from build123d import *

# Parameters (mm, degrees)
SKETCH2_W                 = 230
SKETCH2_H                 = 40
BOSS_EXTRUDE1_DEPTH       = 80
SKETCH6_R                 = 25
BOSS_EXTRUDE3_DEPTH       = 50
SKETCH7_R                 = 12.5
CUT_EXTRUDE2_DEPTH        = 50
SKETCH8_R                 = 26.5
CUT_EXTRUDE3_DEPTH        = 25
CUT_EXTRUDE4_START        = 40
SKETCH11_R                = 26.5
CUT_EXTRUDE4_DEPTH        = 40
SKETCH14_W                = 12.614661349
SKETCH14_H                = 40
CUT_EXTRUDE6_DEPTH        = 50
FILLET3_R                 = 20
FILLET3_OF_MIRROR5_R      = 20
FILLET3_OF_MIRROR8_R      = 20
SKETCH15_W                = 230
SKETCH15_H                = 40
BOSS_EXTRUDE4_DEPTH       = 50
SKETCH18_W                = 206
SKETCH18_H                = 16
CUT_EXTRUDE7_DEPTH        = 80
SKETCH21_R                = 7.5
CUT_EXTRUDE8_DEPTH        = 5
SKETCH22_R                = 5
CUT_EXTRUDE9_DEPTH        = 35
LPATTERN1_COUNT           = 4
LPATTERN1_PITCH           = 17
MIRROR9_COPY_1_SKETCH_R   = 7.5
MIRROR9_COPY_1_DEPTH      = 5
MIRROR9_COPY_2_SKETCH_R   = 7.5
MIRROR9_COPY_2_DEPTH      = 5
MIRROR9_COPY_3_SKETCH_R   = 7.5
MIRROR9_COPY_3_DEPTH      = 5
MIRROR9_COPY_4_SKETCH_R   = 5
MIRROR9_COPY_4_DEPTH      = 35
MIRROR9_COPY_5_SKETCH_R   = 5
MIRROR9_COPY_5_DEPTH      = 35
MIRROR9_COPY_6_SKETCH_R   = 5
MIRROR9_COPY_6_DEPTH      = 35
MIRROR10_COPY_1_SKETCH_R  = 7.5
MIRROR10_COPY_1_DEPTH     = 5
MIRROR10_COPY_2_SKETCH_R  = 7.5
MIRROR10_COPY_2_DEPTH     = 5
MIRROR10_COPY_3_SKETCH_R  = 7.5
MIRROR10_COPY_3_DEPTH     = 5
MIRROR10_COPY_4_SKETCH_R  = 5
MIRROR10_COPY_4_DEPTH     = 35
MIRROR10_COPY_5_SKETCH_R  = 5
MIRROR10_COPY_5_DEPTH     = 35
MIRROR10_COPY_6_SKETCH_R  = 5
MIRROR10_COPY_6_DEPTH     = 35
MIRROR10_COPY_7_SKETCH_R  = 7.5
MIRROR10_COPY_7_DEPTH     = 5
MIRROR10_COPY_8_SKETCH_R  = 5
MIRROR10_COPY_8_DEPTH     = 35
MIRROR10_COPY_9_SKETCH_R  = 7.5
MIRROR10_COPY_9_DEPTH     = 5
MIRROR10_COPY_10_SKETCH_R = 7.5
MIRROR10_COPY_10_DEPTH    = 5
MIRROR10_COPY_11_SKETCH_R = 7.5
MIRROR10_COPY_11_DEPTH    = 5
MIRROR10_COPY_12_SKETCH_R = 5
MIRROR10_COPY_12_DEPTH    = 35
MIRROR10_COPY_13_SKETCH_R = 5
MIRROR10_COPY_13_DEPTH    = 35
MIRROR10_COPY_14_SKETCH_R = 5
MIRROR10_COPY_14_DEPTH    = 35


with BuildPart() as part:
    # Sketch2 → Boss-Extrude1 (new body)
    with BuildSketch(Plane.XY):
        with Locations((115, 20)):
            Rectangle(SKETCH2_W, SKETCH2_H)
    extrude(amount=BOSS_EXTRUDE1_DEPTH)

    # Sketch6 → Boss-Extrude3 (add)
    with BuildSketch(Plane(origin=(140, 0, 0), x_dir=(0, 0, -1), z_dir=(1, 0, 0))):
        with Locations((10, 20)):
            Circle(SKETCH6_R)
    boss_extrude3 = extrude(amount=BOSS_EXTRUDE3_DEPTH)

    # Sketch7 → Cut-Extrude2 (cut)
    with BuildSketch(Plane.ZY.offset(-140)):
        with Locations(Location((-10, 20, 0), (0, 0, 36.869897646))):
            Circle(SKETCH7_R)
    cut_extrude2 = extrude(amount=-CUT_EXTRUDE2_DEPTH, mode=Mode.SUBTRACT)

    # Sketch8 → Cut-Extrude3 (cut)
    with BuildSketch(Plane.ZY.offset(-140)):
        with Locations((-10, 20)):
            Circle(SKETCH8_R)
    cut_extrude3 = extrude(amount=CUT_EXTRUDE3_DEPTH, mode=Mode.SUBTRACT)

    # Sketch11 → Cut-Extrude4 (cut)
    with BuildSketch(Plane(origin=(190, 0, 0), x_dir=(0, 0, -1), z_dir=(1, 0, 0)).offset(CUT_EXTRUDE4_START)):
        with Locations((10, 20)):
            Circle(SKETCH11_R)
    cut_extrude4 = extrude(amount=-CUT_EXTRUDE4_DEPTH, mode=Mode.SUBTRACT)

    # Mirror1: Boss-Extrude3, Cut-Extrude2, Cut-Extrude3, Cut-Extrude4 across plane
    add(boss_extrude3.mirror(Plane(origin=(115, 0, 0), x_dir=(0, 0, 1), z_dir=(1, 0, 0))))
    add(cut_extrude2.mirror(Plane(origin=(115, 0, 0), x_dir=(0, 0, 1), z_dir=(1, 0, 0))), mode=Mode.SUBTRACT)
    add(cut_extrude3.mirror(Plane(origin=(115, 0, 0), x_dir=(0, 0, 1), z_dir=(1, 0, 0))), mode=Mode.SUBTRACT)
    add(cut_extrude4.mirror(Plane(origin=(115, 0, 0), x_dir=(0, 0, 1), z_dir=(1, 0, 0))), mode=Mode.SUBTRACT)

    # Sketch14 → Cut-Extrude6 (cut)
    with BuildSketch(Plane(origin=(90, 0, 0), x_dir=(0, 0, -1), z_dir=(1, 0, 0))):
        with Locations((-13.692669326, 20)):
            Rectangle(SKETCH14_W, SKETCH14_H)
    cut_extrude6 = extrude(amount=CUT_EXTRUDE6_DEPTH, mode=Mode.SUBTRACT)

    # Fillet3
    fillet3_edges = [part.edges().sort_by_distance(p)[0] for p in [
        (115, 40, 20),
        (115, 0, 20),
    ]]
    fillet(fillet3_edges, radius=FILLET3_R - 0.0001)  # a hair under: the kernel refuses the full size

    # Mirror5: Cut-Extrude6 across plane
    add(cut_extrude6.mirror(Plane.ZY.offset(-165)), mode=Mode.SUBTRACT)

    # Fillet3 of Mirror5
    fillet3_of_mirror5_edges = [part.edges().sort_by_distance(p)[0] for p in [
        (210, 40, 20),
        (210, 0, 20),
    ]]
    fillet(fillet3_of_mirror5_edges, radius=FILLET3_OF_MIRROR5_R - 0.0001)  # a hair under: the kernel refuses the full size

    # Mirror8: Cut-Extrude6 across plane
    add(cut_extrude6.mirror(Plane(origin=(65, 0, 0), x_dir=(0, 0, 1), z_dir=(1, 0, 0))), mode=Mode.SUBTRACT)

    # Fillet3 of Mirror8
    fillet3_of_mirror8_edges = [part.edges().sort_by_distance(p)[0] for p in [
        (20, 40, 20),
        (20, 0, 20),
    ]]
    fillet(fillet3_of_mirror8_edges, radius=FILLET3_OF_MIRROR8_R - 0.0001)  # a hair under: the kernel refuses the full size

    # Sketch15 → Boss-Extrude4 (add)
    with BuildSketch(Plane.XY.offset(80)):
        with Locations((115, 20)):
            Rectangle(SKETCH15_W, SKETCH15_H)
    extrude(amount=BOSS_EXTRUDE4_DEPTH)

    # Sketch18 → Cut-Extrude7 (cut)
    with BuildSketch(Plane.XY.offset(130)):
        with Locations((115, 20)):
            Rectangle(SKETCH18_W, SKETCH18_H)
    extrude(amount=-CUT_EXTRUDE7_DEPTH, mode=Mode.SUBTRACT)

    # Sketch21 → Cut-Extrude8 (cut)
    with BuildSketch(Plane(origin=(0, 40, 0), x_dir=(1, 0, 0), z_dir=(0, 1, 0))):
        with Locations(Location((37, -66, 0), (0, 0, 270))):
            Circle(SKETCH21_R)
    cut_extrude8 = extrude(amount=-CUT_EXTRUDE8_DEPTH, mode=Mode.SUBTRACT)

    # Sketch22 → Cut-Extrude9 (cut)
    with BuildSketch(Plane(origin=(0, 35, 0), x_dir=(1, 0, 0), z_dir=(0, 1, 0))):
        with Locations(Location((37, -66, 0), (0, 0, 270))):
            Circle(SKETCH22_R)
    cut_extrude9 = extrude(amount=-CUT_EXTRUDE9_DEPTH, mode=Mode.SUBTRACT)

    # LPattern1: Cut-Extrude8, Cut-Extrude9 ×4
    with Locations(*[(0, 0, i * LPATTERN1_PITCH) for i in range(1, LPATTERN1_COUNT)]):
        add(cut_extrude8, mode=Mode.SUBTRACT)
        add(cut_extrude9, mode=Mode.SUBTRACT)

    # Mirror9: Cut-Extrude8, Cut-Extrude9 across plane
    add(cut_extrude8.mirror(Plane(origin=(63.5, 0, 0), x_dir=(0, 0, 1), z_dir=(1, 0, 0))), mode=Mode.SUBTRACT)
    add(cut_extrude9.mirror(Plane(origin=(63.5, 0, 0), x_dir=(0, 0, 1), z_dir=(1, 0, 0))), mode=Mode.SUBTRACT)

    # Mirror9 copy 1 sketch → Mirror9 copy 1 (cut)
    with BuildSketch(Plane(origin=(127, 40, 17), x_dir=(-1, 0, 0), z_dir=(0, 1, 0))):
        with Locations((37, 66)):
            Circle(MIRROR9_COPY_1_SKETCH_R)
    extrude(amount=-MIRROR9_COPY_1_DEPTH, mode=Mode.SUBTRACT)

    # Mirror9 copy 2 sketch → Mirror9 copy 2 (cut)
    with BuildSketch(Plane(origin=(127, 40, 34), x_dir=(-1, 0, 0), z_dir=(0, 1, 0))):
        with Locations((37, 66)):
            Circle(MIRROR9_COPY_2_SKETCH_R)
    extrude(amount=-MIRROR9_COPY_2_DEPTH, mode=Mode.SUBTRACT)

    # Mirror9 copy 3 sketch → Mirror9 copy 3 (cut)
    with BuildSketch(Plane(origin=(127, 40, 51), x_dir=(-1, 0, 0), z_dir=(0, 1, 0))):
        with Locations((37, 66)):
            Circle(MIRROR9_COPY_3_SKETCH_R)
    extrude(amount=-MIRROR9_COPY_3_DEPTH, mode=Mode.SUBTRACT)

    # Mirror9 copy 4 sketch → Mirror9 copy 4 (cut)
    with BuildSketch(Plane(origin=(127, 35, 17), x_dir=(-1, 0, 0), z_dir=(0, 1, 0))):
        with Locations((37, 66)):
            Circle(MIRROR9_COPY_4_SKETCH_R)
    extrude(amount=-MIRROR9_COPY_4_DEPTH, mode=Mode.SUBTRACT)

    # Mirror9 copy 5 sketch → Mirror9 copy 5 (cut)
    with BuildSketch(Plane(origin=(127, 35, 34), x_dir=(-1, 0, 0), z_dir=(0, 1, 0))):
        with Locations((37, 66)):
            Circle(MIRROR9_COPY_5_SKETCH_R)
    extrude(amount=-MIRROR9_COPY_5_DEPTH, mode=Mode.SUBTRACT)

    # Mirror9 copy 6 sketch → Mirror9 copy 6 (cut)
    with BuildSketch(Plane(origin=(127, 35, 51), x_dir=(-1, 0, 0), z_dir=(0, 1, 0))):
        with Locations((37, 66)):
            Circle(MIRROR9_COPY_6_SKETCH_R)
    extrude(amount=-MIRROR9_COPY_6_DEPTH, mode=Mode.SUBTRACT)

    # Mirror10: Cut-Extrude8, Cut-Extrude9 across plane
    add(cut_extrude8.mirror(Plane(origin=(115, 0, 0), x_dir=(0, 0, 1), z_dir=(1, 0, 0))), mode=Mode.SUBTRACT)
    add(cut_extrude9.mirror(Plane(origin=(115, 0, 0), x_dir=(0, 0, 1), z_dir=(1, 0, 0))), mode=Mode.SUBTRACT)

    # Mirror10 copy 1 sketch → Mirror10 copy 1 (cut)
    with BuildSketch(Plane(origin=(230, 40, 17), x_dir=(-1, 0, 0), z_dir=(0, 1, 0))):
        with Locations((37, 66)):
            Circle(MIRROR10_COPY_1_SKETCH_R)
    extrude(amount=-MIRROR10_COPY_1_DEPTH, mode=Mode.SUBTRACT)

    # Mirror10 copy 2 sketch → Mirror10 copy 2 (cut)
    with BuildSketch(Plane(origin=(230, 40, 34), x_dir=(-1, 0, 0), z_dir=(0, 1, 0))):
        with Locations((37, 66)):
            Circle(MIRROR10_COPY_2_SKETCH_R)
    extrude(amount=-MIRROR10_COPY_2_DEPTH, mode=Mode.SUBTRACT)

    # Mirror10 copy 3 sketch → Mirror10 copy 3 (cut)
    with BuildSketch(Plane(origin=(230, 40, 51), x_dir=(-1, 0, 0), z_dir=(0, 1, 0))):
        with Locations((37, 66)):
            Circle(MIRROR10_COPY_3_SKETCH_R)
    extrude(amount=-MIRROR10_COPY_3_DEPTH, mode=Mode.SUBTRACT)

    # Mirror10 copy 4 sketch → Mirror10 copy 4 (cut)
    with BuildSketch(Plane(origin=(230, 35, 17), x_dir=(-1, 0, 0), z_dir=(0, 1, 0))):
        with Locations((37, 66)):
            Circle(MIRROR10_COPY_4_SKETCH_R)
    extrude(amount=-MIRROR10_COPY_4_DEPTH, mode=Mode.SUBTRACT)

    # Mirror10 copy 5 sketch → Mirror10 copy 5 (cut)
    with BuildSketch(Plane(origin=(230, 35, 34), x_dir=(-1, 0, 0), z_dir=(0, 1, 0))):
        with Locations((37, 66)):
            Circle(MIRROR10_COPY_5_SKETCH_R)
    extrude(amount=-MIRROR10_COPY_5_DEPTH, mode=Mode.SUBTRACT)

    # Mirror10 copy 6 sketch → Mirror10 copy 6 (cut)
    with BuildSketch(Plane(origin=(230, 35, 51), x_dir=(-1, 0, 0), z_dir=(0, 1, 0))):
        with Locations((37, 66)):
            Circle(MIRROR10_COPY_6_SKETCH_R)
    extrude(amount=-MIRROR10_COPY_6_DEPTH, mode=Mode.SUBTRACT)

    # Mirror10 copy 7 sketch → Mirror10 copy 7 (cut)
    with BuildSketch(Plane(origin=(103, 40, 0), x_dir=(1, 0, 0), z_dir=(0, 1, 0))):
        with Locations(Location((37, -66, 0), (0, 0, 270))):
            Circle(MIRROR10_COPY_7_SKETCH_R)
    extrude(amount=-MIRROR10_COPY_7_DEPTH, mode=Mode.SUBTRACT)

    # Mirror10 copy 8 sketch → Mirror10 copy 8 (cut)
    with BuildSketch(Plane(origin=(103, 35, 0), x_dir=(1, 0, 0), z_dir=(0, 1, 0))):
        with Locations(Location((37, -66, 0), (0, 0, 270))):
            Circle(MIRROR10_COPY_8_SKETCH_R)
    extrude(amount=-MIRROR10_COPY_8_DEPTH, mode=Mode.SUBTRACT)

    # Mirror10 copy 9 sketch → Mirror10 copy 9 (cut)
    with BuildSketch(Plane(origin=(103, 40, 17), x_dir=(1, 0, 0), z_dir=(0, 1, 0))):
        with Locations(Location((37, -66, 0), (0, 0, 270))):
            Circle(MIRROR10_COPY_9_SKETCH_R)
    extrude(amount=-MIRROR10_COPY_9_DEPTH, mode=Mode.SUBTRACT)

    # Mirror10 copy 10 sketch → Mirror10 copy 10 (cut)
    with BuildSketch(Plane(origin=(103, 40, 34), x_dir=(1, 0, 0), z_dir=(0, 1, 0))):
        with Locations(Location((37, -66, 0), (0, 0, 270))):
            Circle(MIRROR10_COPY_10_SKETCH_R)
    extrude(amount=-MIRROR10_COPY_10_DEPTH, mode=Mode.SUBTRACT)

    # Mirror10 copy 11 sketch → Mirror10 copy 11 (cut)
    with BuildSketch(Plane(origin=(103, 40, 51), x_dir=(1, 0, 0), z_dir=(0, 1, 0))):
        with Locations(Location((37, -66, 0), (0, 0, 270))):
            Circle(MIRROR10_COPY_11_SKETCH_R)
    extrude(amount=-MIRROR10_COPY_11_DEPTH, mode=Mode.SUBTRACT)

    # Mirror10 copy 12 sketch → Mirror10 copy 12 (cut)
    with BuildSketch(Plane(origin=(103, 35, 17), x_dir=(1, 0, 0), z_dir=(0, 1, 0))):
        with Locations(Location((37, -66, 0), (0, 0, 270))):
            Circle(MIRROR10_COPY_12_SKETCH_R)
    extrude(amount=-MIRROR10_COPY_12_DEPTH, mode=Mode.SUBTRACT)

    # Mirror10 copy 13 sketch → Mirror10 copy 13 (cut)
    with BuildSketch(Plane(origin=(103, 35, 34), x_dir=(1, 0, 0), z_dir=(0, 1, 0))):
        with Locations(Location((37, -66, 0), (0, 0, 270))):
            Circle(MIRROR10_COPY_13_SKETCH_R)
    extrude(amount=-MIRROR10_COPY_13_DEPTH, mode=Mode.SUBTRACT)

    # Mirror10 copy 14 sketch → Mirror10 copy 14 (cut)
    with BuildSketch(Plane(origin=(103, 35, 51), x_dir=(1, 0, 0), z_dir=(0, 1, 0))):
        with Locations(Location((37, -66, 0), (0, 0, 270))):
            Circle(MIRROR10_COPY_14_SKETCH_R)
    extrude(amount=-MIRROR10_COPY_14_DEPTH, mode=Mode.SUBTRACT)


solid = part.part
Work out the finished part from the listing and answer in its coordinate system (mm). A direction names the side the tool comes from. Coordinates: 2 decimals unless noted, no trailing zeros. Order: outer loops, then holes, each group sorted by start corner. A loop starts at its lowest first (then second) coordinate and runs counter-clockwise, first axis right, second up. Notation, with made-up numbers: (89, 20.5) - (134, 20.5) arc R12 cw to (134, 37.5) - close; hole circle Ø5 at (71, 49.5). An arc over 180 degrees is marked (long way). Put each result on its own line as item: value. Start each with the question number.
1) For faces 4 (the cylindrical face through (85.381, 6.084, 81.085)), 5 (the flat face through (135, 35, 85)), 6 (the flat face through (114, 28, 91)), 7 (the cylindrical face through (115.35, 34.297, 26.014)), determine the directions among +Z, -Z, +X, -X, +Y, -Y from which every point of the face is accessible in a straight line to the end or side of a thin tool.
2) For a pull along X with two mould halves and no side action, classify faces 1 (the flat face through (230, 20, 74)), 2 (the cylindrical face through (97.32, 37.53, 64.37)), 3 (the cylindrical face through (209.72, 5.703, 26.014)) as released by +X, released by -X, zero draft, split by the parting line, or undercut.
3) Find section A-A (x = 67). Give the vertices of the cut face in (y, z), plus the area to 3 significant figures.
4) Find the intervals of material crossed by line 1 (X direction, y = 36, z = 19.5); line 2 (Y direction, x = 64.5, z = 81); line 3 (Z direction, x = 193, y = 4), in increasing order. Write a range as from..to.
5) Find section C-C (z = -12.5). Give the vertices of the cut face in (x, y), plus the area to 3 significant figures.
6) Find section B-B (z = 8). Give the vertices of the cut face in (x, y), plus the area to 3 significant figures.
7) Find section D-D (x = 37). State how many separate pieces and enclosed holes the cut face has, plus the area to 3 significant figures.
8) Flat-ended cylindrical pins translate along their axes: pin 1 (8 mm diameter, centred on x = 197.5, z = 6, fed in from -Y); pin 2 (4.5 mm diameter, centred on x = 34.5, z = 80, fed in from +Y); pin 3 (6 mm diameter, centred on y = 4, z = -4, fed in from +X); pin 4 (16.5 mm diameter, centred on x = 196, z = 67.5, fed in from +Y). Find the tip coordinate at first contact, or state that the pin passes through.
Results list:
1. face 4: +Y, -Y
1. face 5: +Y
1. face 6: +Z
1. face 7: -Z, +Y
2. face 1: released by +X
2. face 2: undercut
2. face 3: zero draft
3. outline: (0, 5) arc R25 ccw (long way) to (40, 5) - (40, 130) - (28, 130) - (28, 50) - (12, 50) - (12, 130) - (0, 130) - close; hole circle Ø25 at (20, -10)
3. area: 4,910 mm^2
4. line 1: x = 40..90, 140..190
4. line 2: y = 0..12, 28..40
4. line 3: z = 28..61, 71..78, 88..95, 105..112, 122..130
5. outline: (40, -4.87) - (90, -4.87) - (90, 7.75) - (40, 7.75) - close; (40, 32.25) - (90, 32.25) - (90, 44.87) - (40, 44.87) - close; (140, -4.87) - (190, -4.87) - (190, 7.75) - (140, 7.75) - close; (140, 32.25) - (190, 32.25) - (190, 44.87) - (140, 44.87) - close
5. area: 2,530 mm^2
6. outline: (40, 0) - (90, 0) - (90, 40) - (40, 40) - close; (140, 0) - (190, 0) - (190, 40) - (140, 40) - close
6. area: 4,000 mm^2
7. separate pieces: 9
7. enclosed holes: 0
7. area: 1,890 mm^2
8. pin 1: passes through
8. pin 2: stops at y = 35
8. pin 3: stops at x = 190
8. pin 4: stops at y = 40
